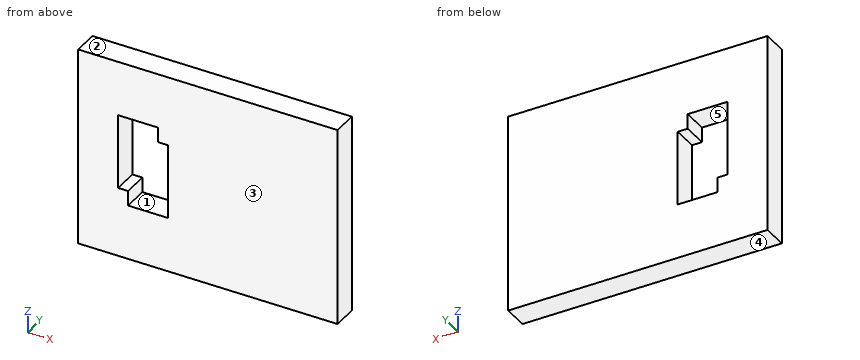
```python
from build123d import *

# Parameters (mm, degrees)
STOCK_895_FRAME_1_START     = 74.5
STOCK_895_FRAME_1_OUTLINE_W = 50
STOCK_895_FRAME_1_OUTLINE_H = 40
STOCK_895_FRAME_1_DEPTH     = 5
SKETCH2_W                   = 5
SKETCH2_H                   = 40
BOSS_EXTRUDE1_DEPTH         = 2


# Read off the part's stored shape, not the designer's step: Stock-895_Frame-1
with BuildPart() as part:
    # Stock-895_Frame-1 outline → Stock-895_Frame-1 (new body)
    with BuildSketch(Plane(origin=(0, 0, 0), x_dir=(1, 0, 0), z_dir=(0, 1, 0)).offset(STOCK_895_FRAME_1_START)):
        with Locations((-25, 0)):
            Rectangle(STOCK_895_FRAME_1_OUTLINE_W, STOCK_895_FRAME_1_OUTLINE_H)
        Polygon((-34, -6), (-34, -9), (-42, -9), (-42, 6), (-40, 6), (-40, 9), (-32, 9), (-32, -6), align=None, mode=Mode.SUBTRACT)
    extrude(amount=STOCK_895_FRAME_1_DEPTH)

    # Sketch2 → Boss-Extrude1 (add)
    with BuildSketch(Plane.YZ):
        with Locations((77, 0)):
            Rectangle(SKETCH2_W, SKETCH2_H)
    extrude(amount=BOSS_EXTRUDE1_DEPTH)


solid = part.part
```
Work out the finished part from the listing and answer in its coordinate system (mm). Face numbers are marked on the shaded views. A direction names the side the tool comes from. Round coordinates to 2 decimals unless told otherwise and drop trailing zeros. Loops run counter-clockwise (first coordinate to the right, second up) from the corner with the lowest first, then second, coordinate; pieces in that order, holes last. Notation, with made-up numbers: M 14,63.5 L 55,63.5 A29 cw 55,89.5 Z; hole C 17,67.25 d4. An arc over 180 degrees is marked long. One line per question, with ' | ' between items.
Q1. Find section B-B, the plane z = 1.5. Give the vertices of the cut face in (x, y), then the cut area to 3 significant figures.
Conclusion:
outline: M -50,74.5 L -42,74.5 L -42,79.5 L -50,79.5 Z; M -32,74.5 L 2,74.5 L 2,79.5 L -32,79.5 Z | area: 210 mm2
Q2. Consider line 1 along X through (y, z) = (79.2, -2.5); line 2 along Z through (x, y) = (-35, 76.7); line 3 along X through (y, z) = (75.75, 7). Determine where each line is inside the solid, lowest interval first. Write a range as from..to.
Conclusion:
line 1: x = -50..-42, -32..2 | line 2: z = -20..-9, 9..20 | line 3: x = -50..-42, -34..2
Q3. Find section A-A, the plane x = -41. Give the vertices of the cut face in (y, z).
Conclusion:
outline: M 74.5,-20 L 79.5,-20 L 79.5,-6 L 74.5,-6 Z; M 74.5,9 L 79.5,9 L 79.5,20 L 74.5,20 Z
Q4. The mould has two halves that part along Z. Classify the marked faces 1, 2 and 3: +Z half, -Z half, draft (parallel to the pull), parting line (faces both ways), or undercut.
Conclusion:
face 1: undercut | face 2: +Z half | face 3: draft
Q5. Find section C-C, the plane y = 78.2. Give the vertices of the cut face in (x, z).
Conclusion:
outline: M -50,-20 L 2,-20 L 2,20 L -50,20 Z; hole M -42,-6 L -40,-6 L -40,-9 L -32,-9 L -32,6 L -34,6 L -34,9 L -42,9 Z
Q6. A tool of negligible diameter and unlimited length cuts with its end or side. For the marked faces 4 and 5, from which of +Z, -Z, +X, -X, +Y, -Y can it reach the whole face along a straight path? Write none if from no direction.
Conclusion:
face 4: -Z, +X, -X, +Y, -Y | face 5: +Y, -Y
